from build123d import *

# Parameters (mm, degrees)
SKETCH1_W           = 34.925
SKETCH1_H           = 6.35
SKETCH1_R           = 1.905
BOSS_EXTRUDE1_DEPTH = 2.54


with BuildPart() as part:
    # Sketch1 → Boss-Extrude1 (new body)
    with BuildSketch(Plane(origin=(0, 0, 0), x_dir=(1, 0, 0), z_dir=(0, 1, 0))):
        with Locations((-4.7625, 0)):
            Rectangle(SKETCH1_W, SKETCH1_H)
        with Locations((-19.05, 0)):
            Circle(SKETCH1_R, mode=Mode.SUBTRACT)
        with Locations((9.525, 0)):
            Circle(SKETCH1_R, mode=Mode.SUBTRACT)
        Circle(SKETCH1_R, mode=Mode.SUBTRACT)
    extrude(amount=BOSS_EXTRUDE1_DEPTH)


solid = part.part
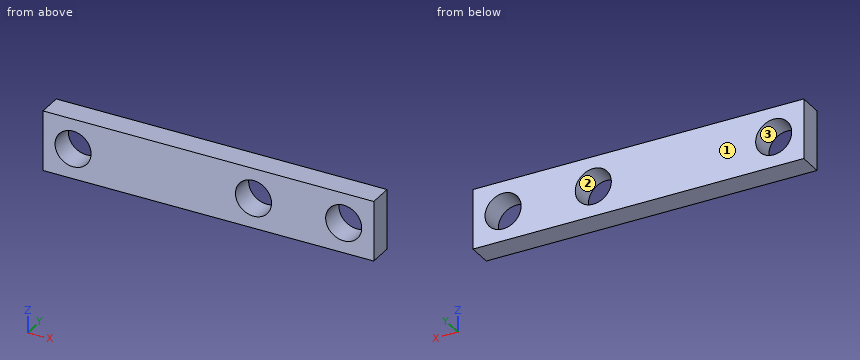
Design review of the part built by this model. Coordinates are the model's own, in mm. Face numbers are marked on the shaded views. Give positions to 0.01 mm unless a question says otherwise; leave off trailing zeros. Loops run counter-clockwise (first coordinate to the right, second up) from the corner with the lowest first, then second, coordinate; pieces in that order, holes last. Notation, with made-up numbers: M -17.75,79.25 L 29.25,79.25 A9 cw 29.25,83.25 Z; hole C -17.5,-11 d9. An arc over 180 degrees is marked long. Answer as a JSON object with one key per item and string values.
Item 1: Mouldability with a two-part tool opening along X and no side actions: class the marked faces 1, 2 and 3 as pulls with the +X half, pulls with the -X half, needs draft (parallel to the pull), parting line crosses it, or undercut.
Output values:
{"face 1": "needs draft", "face 2": "undercut", "face 3": "undercut"}
Item 2: We need section A-A (x = 0). State the section outline as (y, z) points (3 decimals).
Output values:
{"outline": "M 0,-3.175 L 2.54,-3.175 L 2.54,-1.905 L 0,-1.905 Z; M 0,1.905 L 2.54,1.905 L 2.54,3.175 L 0,3.175 Z"}
Item 3: We need section D-D (z = 1.25). State the section outline as (x, y) points (3 decimals).
Output values:
{"outline": "M -22.225,0 L -20.488,0 L -20.488,2.54 L -22.225,2.54 Z; M -17.612,0 L -1.438,0 L -1.438,2.54 L -17.612,2.54 Z; M 1.438,0 L 8.087,0 L 8.087,2.54 L 1.438,2.54 Z; M 10.963,0 L 12.7,0 L 12.7,2.54 L 10.963,2.54 Z"}
Item 4: We need section B-B (z = 0). State the section outline as (x, y) points (3 decimals).
Output values:
{"outline": "M -22.225,0 L -20.955,0 L -20.955,2.54 L -22.225,2.54 Z; M -17.145,0 L -1.905,0 L -1.905,2.54 L -17.145,2.54 Z; M 1.905,0 L 7.62,0 L 7.62,2.54 L 1.905,2.54 Z; M 11.43,0 L 12.7,0 L 12.7,2.54 L 11.43,2.54 Z"}
Item 5: We need section C-C (y = 0.4). State the section outline as (x, z) points (3 decimals).
Output values:
{"outline": "M -22.225,-3.175 L 12.7,-3.175 L 12.7,3.175 L -22.225,3.175 Z; hole C -19.05,0 d3.81; hole C 0,0 d3.81; hole C 9.525,0 d3.81"}
Item 6: Wall thickness on line 1 along X through (y, z) = (2, 0) (3 decimals); line 2 along Z through (x, y) = (-19.05, 2) (3 decimals); line 3 along X through (y, z) = (1.2, -1) (3 decimals): over which ranges is each line inside the solid? List them lowest first.
Output values:
{"line 1": "x = -22.225 to -20.955, -17.145 to -1.905, 1.905 to 7.62, 11.43 to 12.7", "line 2": "z = -3.175 to -1.905, 1.905 to 3.175", "line 3": "x = -22.225 to -20.671, -17.429 to -1.621, 1.621 to 7.904, 11.146 to 12.7"}
